from build123d import *

# Parameters (mm, degrees)
CYLINDER013_R             = 11
CYLINDER013_DEPTH         = 2
CYLINDER014_R             = 2.5
CYLINDER014_DEPTH         = 14
CYLINDER010_R             = 1.5
CYLINDER010_DEPTH         = 10
CYLINDER011_R             = 1.5
CYLINDER011_DEPTH         = 10
CYLINDER012_R             = 1.5
CYLINDER012_DEPTH         = 10
CYLINDER009_R             = 1.5
CYLINDER009_DEPTH         = 10
BOX001_W                  = 39
BOX001_H                  = 31
BOX001_DEPTH              = 39
FUSION001_PLACEMENT_ANGLE = 90


with BuildPart() as cylinder013:
    # Cylinder013 → Cylinder013 (new body)
    with BuildSketch(Plane(origin=(19.5, 33, 19.5), x_dir=(1, 0, 0), z_dir=(0, -1, 0))):
        Circle(CYLINDER013_R)
    extrude(amount=CYLINDER013_DEPTH)


with BuildPart() as cylinder014:
    # Cylinder014 → Cylinder014 (new body)
    with BuildSketch(Plane(origin=(19.5, 33, 19.5), x_dir=(1, 0, 0), z_dir=(0, 1, 0))):
        Circle(CYLINDER014_R)
    extrude(amount=CYLINDER014_DEPTH)


with BuildPart() as cylinder010:
    # Cylinder010 → Cylinder010 (new body)
    with BuildSketch(Plane(origin=(35, 23, 35), x_dir=(1, 0, 0), z_dir=(0, 1, 0))):
        Circle(CYLINDER010_R)
    extrude(amount=CYLINDER010_DEPTH)


with BuildPart() as cylinder011:
    # Cylinder011 → Cylinder011 (new body)
    with BuildSketch(Plane(origin=(35, 23, 4), x_dir=(1, 0, 0), z_dir=(0, 1, 0))):
        Circle(CYLINDER011_R)
    extrude(amount=CYLINDER011_DEPTH)


with BuildPart() as cylinder012:
    # Cylinder012 → Cylinder012 (new body)
    with BuildSketch(Plane(origin=(4, 23, 4), x_dir=(1, 0, 0), z_dir=(0, 1, 0))):
        Circle(CYLINDER012_R)
    extrude(amount=CYLINDER012_DEPTH)


with BuildPart() as cylinder009:
    # Cylinder009 → Cylinder009 (new body)
    with BuildSketch(Plane(origin=(4, 23, 35), x_dir=(1, 0, 0), z_dir=(0, 1, 0))):
        Circle(CYLINDER009_R)
    extrude(amount=CYLINDER009_DEPTH)


with BuildPart() as fusion001:
    # Box001 → Box001 (new body)
    with BuildSketch(Plane.XY):
        with Locations((19.5, 15.5)):
            Rectangle(BOX001_W, BOX001_H)
    extrude(amount=BOX001_DEPTH)

    # Cut005: cut Cylinder009
    add(cylinder009.part, mode=Mode.SUBTRACT)

    # Cut006: cut Cylinder012
    add(cylinder012.part, mode=Mode.SUBTRACT)

    # Cut007: cut Cylinder011
    add(cylinder011.part, mode=Mode.SUBTRACT)

    # Cut008: cut Cylinder010
    add(cylinder010.part, mode=Mode.SUBTRACT)

    # Fusion001: union Cylinder013, Cylinder014
    add(cylinder013.part)
    add(cylinder014.part)


with BuildPart() as fusion001_1:
    # Fusion001 placement: moved
    add(fusion001.part.moved(Location((100, -32.3, 93.7))).rotate(Axis((100, -32.3, 93.7), (-1, 0, 0)), FUSION001_PLACEMENT_ANGLE))


solid = fusion001_1.part
Model file for the job. Use its own axes, mm. A direction names the side the tool comes from. Give positions to 0.01 mm unless a question says otherwise; leave off trailing zeros. Loops run counter-clockwise (first coordinate to the right, second up) from the corner with the lowest first, then second, coordinate; pieces in that order, holes last.
1) Saw through at C-C (z = 55.5). Write the cut outline in (x, y), plus the area to 3 significant figures.
2) Tool access for faces 1 (the flat face through (119, -13, 93.7)), 2 (the flat face through (111, -4, 62.7)): list every direction of +Z, -Z, +X, -X, +Y, -Y with a clear straight run to the whole face (end or side of a thin tool).
3) Saw through at D-D (y = -6). Write the cut outline in (x, z).
4) Wall check: line 1 (Y direction, x = 104, z = 66.75); line 2 (X direction, y = 2, z = 66); line 3 (Z direction, x = 109.5, y = -4). Give the ranges that are in metal, low to high.
5) Saw through at A-A (y = -28.3). Write the cut outline in (x, z), plus the area to 3 significant figures.
6) Saw through at B-B (x = 104). Write the cut outline in (y, z), plus the area to 3 significant figures.
7) Flat gauge pins, fed straight in: pin 1 Ø4 at (x, y) = (108.5, -14.5) entering from -Z; pin 2 Ø0.9 at (x, y) = (104, 2) entering from -Z; pin 3 Ø1 at (x, y) = (127, -3.5) entering from -Z. Where does each tip first touch, or does it go through?
8) Pull direction X, two halves, no side cores. Call faces 3 (the flat face through (135, 3, 70.7)), 4 (the cylindrical face through (121.885, -13.551, 53.798)), 5 (the flat face through (119, -32.3, 78)): +X half, -X half, draft (parallel to the pull), parting line (faces both ways), or undercut.
Answer block:
1. outline: circle Ø5 at (119.5, -12.8)
1. area: 19.6 mm2
2. face 1: +Z, +X, -X, +Y, -Y
2. face 2: -Z
3. outline: (100, 62.7) - (110.85, 62.7) - (110.85, 60.7) - (128.15, 60.7) - (128.15, 62.7) - (139, 62.7) - (139, 93.7) - (100, 93.7) - close
4. line 1: y = -32.3 to -29.8, -26.8 to 1.2, 4.2 to 6.7
4. line 2: x = 100 to 102.67, 105.33 to 133.67, 136.33 to 139
4. line 3: z = 62.7 to 93.7
5. outline: (100, 62.7) - (102.5, 62.7) - (102.5, 70.7) - (105.5, 70.7) - (105.5, 62.7) - (133.5, 62.7) - (133.5, 70.7) - (136.5, 70.7) - (136.5, 62.7) - (139, 62.7) - (139, 93.7) - (100, 93.7) - close
5. area: 1,160 mm2
6. outline: (-32.3, 62.7) - (-29.8, 62.7) - (-29.8, 70.7) - (-26.8, 70.7) - (-26.8, 62.7) - (1.2, 62.7) - (1.2, 70.7) - (4.2, 70.7) - (4.2, 62.7) - (6.7, 62.7) - (6.7, 93.7) - (-32.3, 93.7) - close
6. area: 1,160 mm2
7. pin 1: stops at z = 60.7
7. pin 2: stops at z = 70.7
7. pin 3: stops at z = 62.7
8. face 3: undercut
8. face 4: parting line
8. face 5: draft
